Answer from the drawing. Dimensions are ordinates in mm from the lowest x, y and z of the part. Coordinates: 2 decimals unless noted, no trailing zeros. Write each loop counter-clockwise with the first axis right and the second up, starting at its lowest first coordinate (ties: lowest second). Pieces come first, ordered by that corner, then holes. Notation, with made-up numbers: (45, 47) - (95, 47) arc R24 ccw to (95, 63) - close; hole circle Ø10 at (-5, 56.5). An arc over 180 degrees is marked (long way). Return JSON: item names as keys, results as strings.
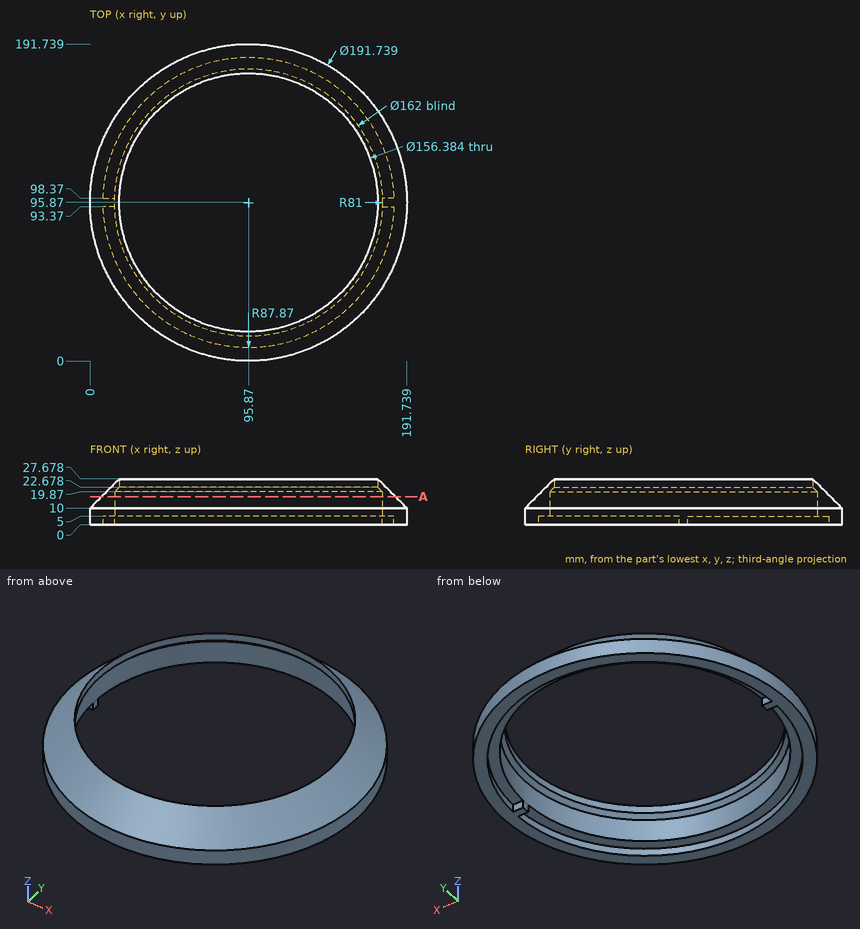
(1) Straight lines are drawn through the part: line 1 (Y direction, x = 119, z = 4.5); line 2 (Y direction, x = 30, z = 12.75); line 3 (X direction, y = 143.5, z = 6) (1 decimal). For each, find the intervals that lie inside material, in ascending order. Write a range as from..to.
Answer:
{"line 1": "2.83..11.1, 180.64..188.91", "line 2": "30.05..48.73, 143.01..161.69", "line 3": "12.7..30.4, 161.4..179.1"}
(2) Flat-ended cylindrical pins translate along their axes: P1, Ø1, axis at x = 56, z = 7.5, coming from the +Y side; P2, Ø4, axis at x = 179.5, z = 2, coming from the +Y side (1 decimal); P3, Ø1.5, axis at x = 181, z = 3, coming from the -Y side. Find the tip coordinate at first contact, or state that the pin passes through.
Answer:
{"P1": "y = 183.28", "P2": "y = 146.1", "P3": "y = 50.36"}
(3) A cutting plane is placed at A-A (z = 17). Determine the outline of the cut face in (x, y).
Answer:
{"outline": "circle Ø177.74 at (95.87, 95.87); hole circle Ø162 at (95.87, 95.87)"}
